from build123d import *

# Parameters (mm, degrees)
M4_CLEARANCE_HOLE1_D   = 4.5
CUT_EXTRUDE1_START     = -24
CUT_EXTRUDE1_OUTLINE_R = 2.25
CUT_EXTRUDE1_DEPTH     = 26
SKETCH8_R              = 2.25
CUT_EXTRUDE2_DEPTH     = 26


# Read off the part's stored shape, not the designer's step: Cut-Extrude1
with BuildPart() as part:
    # Sweep1: sweep along a path in Sketch1
    with BuildLine(Plane(origin=(0, 152.68757152, 0), x_dir=(1, 0, 0), z_dir=(0, 1, 0))) as sweep1_path:
        Line((77.38365074, -11.079514347), (77.38365074, -91.079514347))
        ThreePointArc((77.38365074, -91.079514347), (63.83733937, -123.783202977), (31.13365074, -137.329514347))
        Line((31.13365074, -137.329514347), (-46.36634926, -137.329514347))
        ThreePointArc((-46.36634926, -137.329514347), (-79.07003789, -123.783202977), (-92.61634926, -91.079514347))
        Line((-92.61634926, -91.079514347), (-92.61634926, -23.579514347))
        ThreePointArc((-92.61634926, -23.579514347), (-79.07003789, 9.124174283), (-46.36634926, 22.670485653))
        Line((-46.36634926, 22.670485653), (-16.36634926, 22.670485653))
    # Sketch2 → Sweep1 (sweep)
    with BuildSketch(Plane.ZY.offset(52.61634926)):
        Polygon((-25.670485653, 153.211679549), (-25.670485653, 158.68757152), (-19.670485653, 158.68757152), (-19.670485653, 148.68757152), (-19.670485653, 142.68757152), (-19.670485653, 122.68757152), (-25.670485653, 122.68757152), (-25.670485653, 142.68757152), align=None)
    sweep(path=sweep1_path.line)

    # M4 Clearance Hole1 (through all)
    with Locations(Plane(origin=(0, 158.68757152, 0), x_dir=(1, 0, 0), z_dir=(0, 1, 0))):
        with Locations((-22.61634926, 22.670485653), (77.38365074, -17.329514347)):
            Hole(M4_CLEARANCE_HOLE1_D / 2)

    # Cut-Extrude1 outline → Cut-Extrude1 (cut)
    # profile 1 of 2: a face of its own
    with BuildSketch(Plane(origin=(0, 148.68757152, 0), x_dir=(1, 0, 0), z_dir=(0, 1, 0)).offset(CUT_EXTRUDE1_START)):
        Polygon((74.831520752, -51.329514347), (80.776483816, -51.329514347), (80.776483816, -11.542249894), (74.831520752, -10.731439084), align=None)
        with Locations((77.38365074, -17.329514347)):
            Circle(CUT_EXTRUDE1_OUTLINE_R, mode=Mode.SUBTRACT)
    # profile 2 of 2: a face of its own
    with BuildSketch(Plane(origin=(0, 148.68757152, 0), x_dir=(1, 0, 0), z_dir=(0, 1, 0)).offset(CUT_EXTRUDE1_START)):
        with BuildLine():
            ThreePointArc((-45.903613713, 26.063318729), (-49.266640093, 25.980684534), (-52.61634926, 25.670485653))
            Line((-52.61634926, 25.670485653), (-52.61634926, 19.670485653))
            ThreePointArc((-52.61634926, 19.670485653), (-49.672978387, 19.99445958), (-46.714424523, 20.118355665))
            Line((-46.714424523, 20.118355665), (-16.714424523, 20.118355665))
            Line((-16.714424523, 20.118355665), (-15.903613713, 26.063318729))
            Line((-15.903613713, 26.063318729), (-45.903613713, 26.063318729))
        make_face()
        with Locations((-42.61634926, 22.670485653)):
            Circle(CUT_EXTRUDE1_OUTLINE_R, mode=Mode.SUBTRACT)
        with Locations((-22.61634926, 22.670485653)):
            Circle(CUT_EXTRUDE1_OUTLINE_R, mode=Mode.SUBTRACT)
    extrude(amount=CUT_EXTRUDE1_DEPTH, mode=Mode.SUBTRACT)

    # Sketch8 → Cut-Extrude2 (cut)
    with BuildSketch(Plane(origin=(0, 124.68757152, 0), x_dir=(1, 0, 0), z_dir=(0, 1, 0))):
        with Locations(Location((-22.61634926, 22.670485653, 0), (0, 0, 270))):
            Circle(SKETCH8_R)
        with Locations((-42.61634926, 22.670485653)):
            Circle(SKETCH8_R)
    extrude(amount=CUT_EXTRUDE2_DEPTH, mode=Mode.SUBTRACT)


solid = part.part
Source: CAD feature listing. Evaluate the final solid. Frame: model axes, mm. A direction names the side the tool comes from. Coordinates: 2 decimals unless noted, no trailing zeros. Loops run counter-clockwise (first coordinate to the right, second up) from the corner with the lowest first, then second, coordinate; pieces in that order, holes last. Notation, with made-up numbers: (23, 38.25) - (82, 38.25) arc R22 ccw to (82, 73.25) - close; hole circle Ø2 at (1.25, 60). An arc over 180 degrees is marked (long way). One line per item, written item: value. Start each with the question number.
1. Section C-C (z = 35.5). Return the cut outline in (x, y).
2. Ray query, L1, parallel to X at y = 135, z = 84; L2, parallel to Z at x = -42, y = 138; L3, parallel to X at y = 137, z = 44. Return the intervals inside material, ascending.
3. Mould query, pull axis X, two halves, no side actions, for faces 1 (the flat face through (-96.009, 141, 56)), 2 (the flat face through (78, 124.688, 31)), 3 (the cylindrical face through (77.871, 123.674, 19.526)). Classes: pulls with the +X half, pulls with the -X half, needs draft (parallel to the pull), parting line crosses it, or undercut.
4. Set-up query: faces 4 (the flat face through (-16.315, 154.632, -23.049)), 5 (the flat face through (-31, 155, -26.063)), 6 (the flat face through (78, 150.688, 31)), 7 (the cylindrical face through (-76.675, 140.94, 122.56)). Return all of +Z, -Z, +X, -X, +Y, -Y with unobstructed straight access to the full face (end or side cutting, diameter ignored); none if empty.
5. Section A-A (z = 56). Return the cut outline in (x, y), and give its area (3 significant figures).
6. Contact query for flat-ended pins moving along their axis: P1, Ø1, axis at x = -27, y = 123.5, coming from the +Z side; P2, Ø1.5, axis at y = 142.5, z = 96.5, coming from the +X side; P3, Ø9, axis at x = -26, y = 155.5, coming from the -Z side. Output: stop coordinate, or through.
7. Section D-D (x = -74.5). Return the cut outline in (y, z), and give its area (3 significant figures).
8. Section B-B (x = -37.5). Return the cut outline in (y, z), and give its area (3 significant figures).
Verdict:
1. outline: (-96.01, 122.69) - (-90.06, 122.69) - (-90.06, 158.69) - (-96.01, 158.69) - close; (74.83, 122.69) - (80.78, 122.69) - (80.78, 124.69) - (74.83, 124.69) - close; (74.83, 150.69) - (80.78, 150.69) - (80.78, 158.69) - (74.83, 158.69) - close
2. L1: x = -96.01 to -90.06, 74.83 to 80.78
2. L2: z = 134.78 to 140.72
2. L3: x = -96.01 to -90.06
3. face 1: pulls with the -X half
3. face 2: needs draft
3. face 3: undercut
4. face 4: +X, +Y, -Y
4. face 5: -Z, +X, -X, +Y, -Y
4. face 6: -Z, +X
4. face 7: +Y, -Y
5. outline: (-96.01, 122.69) - (-90.06, 122.69) - (-90.06, 158.69) - (-96.01, 158.69) - close; (74.83, 122.69) - (80.78, 122.69) - (80.78, 158.69) - (74.83, 158.69) - close
5. area: 428 mm2
6. P1: stops at z = 140.72
6. P2: stops at x = 80.56
6. P3: stops at z = -26.06
7. outline: (122.69, -17.32) - (158.69, -17.32) - (158.69, -9.86) - (122.69, -9.86) - close; (122.69, 124.52) - (158.69, 124.52) - (158.69, 131.98) - (122.69, 131.98) - close
7. area: 538 mm2
8. outline: (122.69, -26.06) - (124.69, -26.06) - (124.69, -20.12) - (122.69, -20.12) - close; (122.69, 134.78) - (158.69, 134.78) - (158.69, 140.72) - (122.69, 140.72) - close; (150.69, -26.06) - (158.69, -26.06) - (158.69, -20.12) - (150.69, -20.12) - close
8. area: 273 mm2
